Answer from the drawing. Dimensions are ordinates in mm from the lowest x, y and z of the part. A direction names the side the tool comes from. Give positions to 0.01 mm unless a question says otherwise; leave off trailing zeros. Order: outer loops, then holes, each group sorted by start corner. A loop starts at its lowest first (then second) coordinate and runs counter-clockwise, first axis right, second up.
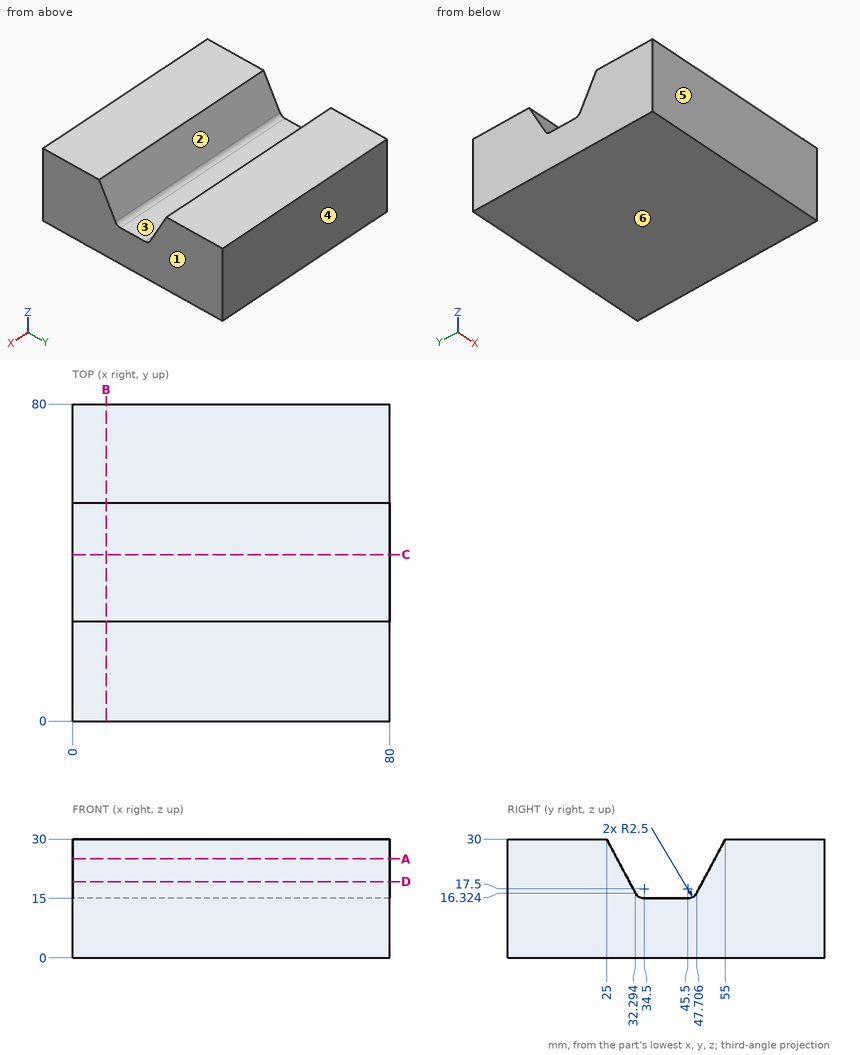
1. The part is cut by section D-D (z = 19.25). Write down the section's boundary in (x, y).
Findings below:
outline: (0, 0) - (80, 0) - (80, 30.73) - (0, 30.73) - close; (0, 49.27) - (80, 49.27) - (80, 80) - (0, 80) - close
2. Given P1, Ø6, axis at x = 31.5, y = 43.5, coming from the +Z side; P2, Ø8, axis at y = 33, z = 20.5, coming from the -X side; P3, Ø3.5, axis at x = 40, y = 38.5, coming from the +Z side, each flat-ended and moving along its own axis, determine where each tip first touches the part or whether it passes through.
Findings below:
P1: stops at z = 15.21
P2: stops at x = 0
P3: stops at z = 15
3. The part is cut by section A-A (z = 25). Write down the section's boundary in (x, y).
Findings below:
outline: (0, 0) - (80, 0) - (80, 27.67) - (0, 27.67) - close; (0, 52.33) - (80, 52.33) - (80, 80) - (0, 80) - close
4. The part is cut by section C-C (y = 42). Write down the section's boundary in (x, z).
Findings below:
outline: (0, 0) - (80, 0) - (80, 15) - (0, 15) - close
5. The mould has two halves that part along Y. Classify the marked faces 3, 4, 5 and 6: pulls with the +Y half, pulls with the -Y half, needs draft (parallel to the pull), parting line crosses it, or undercut.
Findings below:
face 3: undercut
face 4: pulls with the +Y half
face 5: pulls with the -Y half
face 6: needs draft
6. Which of the six approach directions +Z, -Z, +X, -X, +Y, -Y give full straight-line access (tool end or side, diameter ignored) to the marked faces 1 and 2?
Findings below:
face 1: +Z, -Z, +X, +Y, -Y
face 2: +Z, +X, -X
7. Straight lines are drawn through the part: probe 1 along Y at (x, z) = (31.5, 24.25) (1 decimal); probe 2 along Y at (x, z) = (55, 23.75) (1 decimal); probe 3 along Z at (x, y) = (39, 36.5). For each, find the intervals that lie inside material, in ascending order.
Findings below:
probe 1: y = 0 to 28.1, 51.9 to 80
probe 2: y = 0 to 28.3, 51.7 to 80
probe 3: z = 0 to 15
8. The part is cut by section B-B (x = 8.5). Write down the section's boundary in (y, z) (1 decimal), then the cut area to 3 significant figures.
Findings below:
outline: (0, 0) - (80, 0) - (80, 30) - (55, 30) - (47.7, 16.3) arc R2.5 cw to (45.5, 15) - (34.5, 15) arc R2.5 cw to (32.3, 16.3) - (25, 30) - (0, 30) - close
area: 2,070 mm2
